```python
from build123d import *

# Parameters (mm, degrees)
FILLET1_R           = 0.6
FILLET2_R           = 0.6
SQRDRVSKE_OUTSIDE_W = 34.706
SQRDRVSKE_OUTSIDE_H = 34.706
SQUARE_DRIVE_DEPTH  = 12


with BuildPart() as part:
    # BodySke → Base-Revolve (revolve)
    with BuildSketch(Plane.XY, mode=Mode.PRIVATE) as base_revolve_sk:
        Polygon((0, 0), (0, 9.75), (15, 9.75), (15, 6), (59.036, 6), (60, 5.036), (60, 0), align=None)
    revolve(base_revolve_sk.sketch.rotate(Axis((-31.75, 0, 0), (1, 0, 0)), 90), axis=Axis((-31.75, 0, 0), (1, 0, 0)))

    # Fillet1
    fillet1_edges = [part.edges().sort_by_distance(p)[0] for p in [
        (15, 0, -6),
    ]]
    fillet(fillet1_edges, radius=FILLET1_R)

    # Fillet2
    fillet2_edges = [part.edges().sort_by_distance(p)[0] for p in [
        (0, 0, -9.75),
    ]]
    fillet(fillet2_edges, radius=FILLET2_R)

    # SqrDrvSke outside → Square drive (cut)
    with BuildSketch(Plane(origin=(0, 0, 0), x_dir=(0, 0, -1), z_dir=(1, 0, 0))):
        Rectangle(SQRDRVSKE_OUTSIDE_W, SQRDRVSKE_OUTSIDE_H)
        with BuildLine():
            Line((1.950442767, -7.241945389), (7.241945389, -1.950442767))
            ThreePointArc((7.241945389, -1.950442767), (7.5, 0), (7.241945389, 1.950442767))
            Line((7.241945389, 1.950442767), (1.950442767, 7.241945389))
            ThreePointArc((1.950442767, 7.241945389), (0, 7.5), (-1.950442767, 7.241945389))
            Line((-1.950442767, 7.241945389), (-7.241945389, 1.950442767))
            ThreePointArc((-7.241945389, 1.950442767), (-7.5, 0), (-7.241945389, -1.950442767))
            Line((-7.241945389, -1.950442767), (-1.950442767, -7.241945389))
            ThreePointArc((-1.950442767, -7.241945389), (0, -7.5), (1.950442767, -7.241945389))
        make_face(mode=Mode.SUBTRACT)
    extrude(amount=SQUARE_DRIVE_DEPTH, mode=Mode.SUBTRACT)


solid = part.part
```
Could you check a few things on this model? Use its own coordinates, in mm. A direction names the side the tool comes from. Round coordinates to 2 decimals unless told otherwise and drop trailing zeros. Write each loop counter-clockwise with the first axis right and the second up, starting at its lowest first coordinate (ties: lowest second). Pieces come first, ordered by that corner, then holes. Notation, with made-up numbers: M 35,75.25 L 60,75.25 A20 cw 60,79.25 Z; hole C 18.5,-25 d7. An arc over 180 degrees is marked long. Write each question's results on one line, items separated by ' | '. Start each with the question number.
1. Imagine slicing it at C-C on x = 45. List the corners of the cut face in (y, z) for me.
2. On a 3-axis mill with a long thin cutter (end or side, diameter ignored), from which of +Z, -Z, +X, -X, +Y, -Y can I reach the whole of each face in a straight line? I mean faces 1 (the face through (5.92, -4.56, 4.63)), 2 (the face through (5.9, 0, 7.5)), 3 (the face through (5.9, -7.5, 0)), 4 (the face through (5.9, 7.5, 0)). Say none if no direction works.
3. I'm going to push flat-ended pins straight in: pin 1 Ø3 at (x, z) = (43.5, -7) entering from +Y; pin 2 Ø6 at (x, z) = (46, -6.5) entering from +Y; pin 3 Ø1 at (x, z) = (22.5, -1.5) entering from +Y. Where does each tip first touch, or does it pass through?
4. Imagine slicing it at A-A on y = 0. List the corners of the cut face in (x, z) for me, and give its area (3 significant figures).
5. I need wall thicknesses on L1, parallel to X at y = -6.5, z = -5; L2, parallel to Y at x = 15.5, z = 0.25; L3, parallel to Z at x = 35, y = -0.25. Which ranges of each line are inside material? Lowest first, please. Write a range as from..to.
Result sheet:
1) outline: C 0,0 d12
2) face 1: +Z, -X, -Y | face 2: +Z, -X | face 3: -X, -Y | face 4: -X, +Y
3) pin 1: stops at y = 2.4 | pin 2: stops at y = 4.87 | pin 3: stops at y = 5.92
4) outline: M 0,-7.5 L 12,-7.5 L 12,-9.75 L 15,-9.75 L 15,-6.6 A0.6 cw 15.6,-6 L 59.04,-6 L 60,-5.04 L 60,5.04 L 59.04,6 L 15.6,6 A0.6 cw 15,6.6 L 15,9.75 L 12,9.75 L 12,7.5 L 0,7.5 Z | area: 778 mm^2
5) L1: x = 12..15 | L2: y = -6..6 | L3: z = -5.99..5.99
